```python
from build123d import *

# Parameters (mm, degrees)
SKETCH_R      = 60
SKETCH_R_2    = 25.7
SKETCH_R_3    = 1.75
PAD_DEPTH     = 2.2
SKETCH001_R   = 54.2
SKETCH001_R_2 = 51.4
SKETCH001_R_3 = 2.9
SKETCH001_R_4 = 1.65
PAD001_DEPTH  = 5


with BuildPart() as part:
    # Sketch → Pad (new body)
    with BuildSketch(Plane.XY):
        Circle(SKETCH_R)
        Circle(SKETCH_R_2, mode=Mode.SUBTRACT)
        with Locations((0, 47.75)):
            Circle(SKETCH_R_3, mode=Mode.SUBTRACT)
        with Locations((33.764349, 33.764349)):
            Circle(SKETCH_R_3, mode=Mode.SUBTRACT)
        with Locations((47.75, 0)):
            Circle(SKETCH_R_3, mode=Mode.SUBTRACT)
        with Locations((33.764349, -33.764349)):
            Circle(SKETCH_R_3, mode=Mode.SUBTRACT)
        with Locations((0, -47.75)):
            Circle(SKETCH_R_3, mode=Mode.SUBTRACT)
        with Locations((-33.764349, -33.764349)):
            Circle(SKETCH_R_3, mode=Mode.SUBTRACT)
        with Locations((-47.75, 0)):
            Circle(SKETCH_R_3, mode=Mode.SUBTRACT)
        with Locations((-33.764349, 33.764349)):
            Circle(SKETCH_R_3, mode=Mode.SUBTRACT)
    extrude(amount=PAD_DEPTH)

    # Sketch001 → Pad001 (join)
    with BuildSketch(Plane.XY):
        Circle(SKETCH001_R)
        Circle(SKETCH001_R_2, mode=Mode.SUBTRACT)
        with Locations((0, 47)):
            Circle(SKETCH001_R_3)
        with Locations((0, 47)):
            Circle(SKETCH001_R_4, mode=Mode.SUBTRACT)
        with Locations((33.234019, 33.234019)):
            Circle(SKETCH001_R_3)
        with Locations((33.234019, 33.234019)):
            Circle(SKETCH001_R_4, mode=Mode.SUBTRACT)
        with Locations((47, 0)):
            Circle(SKETCH001_R_3)
        with Locations((47, 0)):
            Circle(SKETCH001_R_4, mode=Mode.SUBTRACT)
        with Locations((33.234019, -33.234019)):
            Circle(SKETCH001_R_3)
        with Locations((33.234019, -33.234019)):
            Circle(SKETCH001_R_4, mode=Mode.SUBTRACT)
        with Locations((0, -47)):
            Circle(SKETCH001_R_3)
        with Locations((0, -47)):
            Circle(SKETCH001_R_4, mode=Mode.SUBTRACT)
        with Locations((-33.234019, -33.234019)):
            Circle(SKETCH001_R_3)
        with Locations((-33.234019, -33.234019)):
            Circle(SKETCH001_R_4, mode=Mode.SUBTRACT)
        with Locations((-47, 0)):
            Circle(SKETCH001_R_3)
        with Locations((-47, 0)):
            Circle(SKETCH001_R_4, mode=Mode.SUBTRACT)
        with Locations((-33.234019, 33.234019)):
            Circle(SKETCH001_R_3)
        with Locations((-33.234019, 33.234019)):
            Circle(SKETCH001_R_4, mode=Mode.SUBTRACT)
    extrude(amount=PAD001_DEPTH)


solid = part.part
```
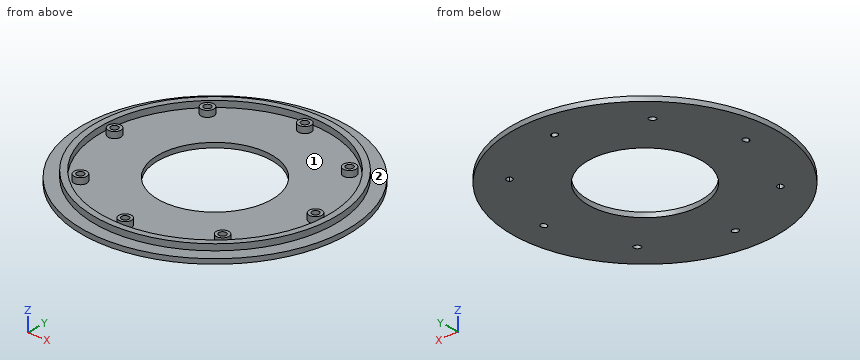
Input: part model. Units: mm. Frame: model coordinates. Face numbers are marked on the shaded views. Coordinates: 2 decimals unless noted, no trailing zeros. Order: outer loops, then holes, each group sorted by start corner. A loop starts at its lowest first (then second) coordinate and runs counter-clockwise, first axis right, second up. Notation, with made-up numbers: (18.5, -0.75) - (25.5, -0.75) arc R10 cw to (25.5, 9.25) - close; hole circle Ø5 at (47.25, 39). An arc over 180 degrees is marked (long way). Return JSON: item names as keys, results as strings.
Q1. Cut plane D-D (x = -21.5). Return loops of the section in (y, z), then the cut area to 3 significant figures.
The answers:
{"outline": "(-56.02, 0) - (-14.08, 0) - (-14.08, 2.2) - (-46.69, 2.2) - (-46.69, 5) - (-49.75, 5) - (-49.75, 2.2) - (-56.02, 2.2) - close; (14.08, 0) - (56.02, 0) - (56.02, 2.2) - (49.75, 2.2) - (49.75, 5) - (46.69, 5) - (46.69, 2.2) - (14.08, 2.2) - close", "area": "202 mm2"}
Q2. First-contact query: pin 1 (3 mm diameter, centred on x = 33.23, y = -33.23, fed in from +Z); pin 2 (1.5 mm diameter, centred on y = 21.5, z = 2.5, fed in from -X); pin 3 (1 mm diameter, centred on x = 7, z = 2, fed in from +Y); pin 4 (0.9 mm diameter, centred on x = -46.5, y = 0, fed in from +Z) (1 decimal). Flat tips, straight axial feed; report the tip coordinate or a pass-through.
The answers:
{"pin 1": "stops at z = 2.2", "pin 2": "stops at x = -56.27", "pin 3": "stops at y = 59.65", "pin 4": "passes through"}
Q3. Cut plane A-A (z = 3.7). State how many separate pieces and enclosed holes the cut face has, then the cut area to 3 significant figures.
The answers:
{"separate pieces": "9", "enclosed holes": "9", "area": "1,070 mm2"}
Q4. Cut plane B-B (y = 7). Return loops of the section in (x, z), then the cut area to 3 significant figures.
The answers:
{"outline": "(-59.59, 0) - (-24.73, 0) - (-24.73, 2.2) - (-50.92, 2.2) - (-50.92, 5) - (-53.75, 5) - (-53.75, 2.2) - (-59.59, 2.2) - close; (24.73, 0) - (59.59, 0) - (59.59, 2.2) - (53.75, 2.2) - (53.75, 5) - (50.92, 5) - (50.92, 2.2) - (24.73, 2.2) - close", "area": "169 mm2"}
Q5. Draft query along Y for the marked faces 1 and 2. Return one class per face: +Y half, -Y half, draft (parallel to the pull), parting line (faces both ways), or undercut.
The answers:
{"face 1": "undercut", "face 2": "draft"}
Q6. Ray query, probe 1 along Y at (x, z) = (0, 3.8); probe 2 along X at (y, z) = (47, 3.2); probe 3 along Y at (x, z) = (-33, 0.8). Return the intervals inside material, ascending.
The answers:
{"probe 1": "y = -54.2 to -51.4, -49.9 to -48.65, -45.35 to -44.1, 44.1 to 45.35, 48.65 to 49.9, 51.4 to 54.2", "probe 2": "x = -26.99 to -20.81, -2.9 to -1.65, 1.65 to 2.9, 20.81 to 26.99", "probe 3": "y = -50.11 to -34.87, -32.19 to 32.19, 34.87 to 50.11"}
